Design review of the part built by this model. Coordinates are the model's own, in mm. Face numbers are marked on the shaded views. A direction names the side the tool comes from. Coordinates: 2 decimals unless noted, no trailing zeros. Write each loop counter-clockwise with the first axis right and the second up, starting at its lowest first coordinate (ties: lowest second). Pieces come first, ordered by that corner, then holes. Notation, with made-up numbers: (-20.5, 42.5) - (3.5, 42.5) arc R31 ccw to (3.5, 80.5) - close; hole circle Ø9 at (25.25, -25.75). An arc over 180 degrees is marked (long way). Answer as a JSON object with one key per item and string values.
```python
from build123d import *

# Parameters (mm, degrees)
F1_DEPTH      = 10
F1_DEPTH_BACK = 10
F2_R          = 4.5
F3_DEPTH      = 4
F4_R          = 3.5
F5_DEPTH      = 25.2476


with BuildPart() as f1:
    # F0 (on Front) → F1 (new body, two sides)
    with BuildSketch(Plane.XZ) as f1_sk:
        with BuildLine():
            ThreePointArc((4.518019, -1.1), (4.616887, -0.553945), (4.65, 0))
            ThreePointArc((4.65, 0), (4.616887, 0.553945), (4.518019, 1.1))
            ThreePointArc((4.518019, 1.1), (4.422413, 1.436929), (4.301718, 1.765707))
            ThreePointArc((4.301718, 1.765707), (3.761929, 2.733201), (3.008591, 3.545544))
            ThreePointArc((3.008591, 3.545544), (2.733201, 3.761929), (2.442307, 3.956973))
            ThreePointArc((2.442307, 3.956973), (1.436929, 4.422413), (0.349983, 4.636811))
            ThreePointArc((0.349983, 4.636811), (0, 4.65), (-0.349983, 4.636811))
            ThreePointArc((-0.349983, 4.636811), (-1.436929, 4.422413), (-2.442307, 3.956973))
            ThreePointArc((-2.442307, 3.956973), (-2.733201, 3.761929), (-3.008591, 3.545544))
            ThreePointArc((-3.008591, 3.545544), (-3.761929, 2.733201), (-4.301718, 1.765707))
            ThreePointArc((-4.301718, 1.765707), (-4.422413, 1.436929), (-4.518019, 1.1))
            ThreePointArc((-4.518019, 1.1), (-4.65, 0), (-4.518019, -1.1))
            ThreePointArc((-4.518019, -1.1), (-4.422413, -1.436929), (-4.301718, -1.765707))
            ThreePointArc((-4.301718, -1.765707), (-3.761929, -2.733201), (-3.008591, -3.545544))
            ThreePointArc((-3.008591, -3.545544), (-2.733201, -3.761929), (-2.442307, -3.956973))
            ThreePointArc((-2.442307, -3.956973), (-1.436929, -4.422413), (-0.349983, -4.636811))
            ThreePointArc((-0.349983, -4.636811), (0, -4.65), (0.349983, -4.636811))
            ThreePointArc((0.349983, -4.636811), (1.436929, -4.422413), (2.442307, -3.956973))
            ThreePointArc((2.442307, -3.956973), (2.733201, -3.761929), (3.008591, -3.545544))
            ThreePointArc((3.008591, -3.545544), (3.761929, -2.733201), (4.301718, -1.765707))
            ThreePointArc((4.301718, -1.765707), (4.422413, -1.436929), (4.518019, -1.1))
        make_face()
        with BuildLine():
            ThreePointArc((4.518019, 1.1), (4.616887, 0.553945), (4.65, 0))
            ThreePointArc((4.65, 0), (4.616887, -0.553945), (4.518019, -1.1))
            Line((4.518019, -1.1), (4.618019, -1.1))
            Line((4.618019, -1.1), (6.25, -0.329923))
            Line((6.25, -0.329923), (6.25, 0))
            Line((6.25, 0), (6.25, 0.329923))
            Line((6.25, 0.329923), (4.618019, 1.1))
            Line((4.618019, 1.1), (4.518019, 1.1))
        make_face()
        with BuildLine():
            ThreePointArc((3.008591, 3.545544), (3.761929, 2.733201), (4.301718, 1.765707))
            Line((4.301718, 1.765707), (4.38262, 1.824485))
            Line((4.38262, 1.824485), (5.25028, 3.406744))
            Line((5.25028, 3.406744), (5.056356, 3.673658))
            Line((5.056356, 3.673658), (4.862432, 3.940572))
            Line((4.862432, 3.940572), (3.089492, 3.604322))
            Line((3.089492, 3.604322), (3.008591, 3.545544))
        make_face()
        with BuildLine():
            Line((4.38262, -1.824485), (4.301718, -1.765707))
            ThreePointArc((4.301718, -1.765707), (3.761929, -2.733201), (3.008591, -3.545544))
            Line((3.008591, -3.545544), (3.089492, -3.604322))
            Line((3.089492, -3.604322), (4.862432, -3.940572))
            Line((4.862432, -3.940572), (5.056356, -3.673658))
            Line((5.056356, -3.673658), (5.25028, -3.406744))
            Line((5.25028, -3.406744), (4.38262, -1.824485))
        make_face()
        with BuildLine():
            ThreePointArc((0.349983, 4.636811), (1.436929, 4.422413), (2.442307, 3.956973))
            Line((2.442307, 3.956973), (2.473209, 4.052079))
            Line((2.473209, 4.052079), (2.245132, 5.842151))
            Line((2.245132, 5.842151), (1.931356, 5.944103))
            Line((1.931356, 5.944103), (1.61758, 6.046055))
            Line((1.61758, 6.046055), (0.380884, 4.731916))
            Line((0.380884, 4.731916), (0.349983, 4.636811))
        make_face()
        with BuildLine():
            Line((2.473209, -4.052079), (2.442307, -3.956973))
            ThreePointArc((2.442307, -3.956973), (1.436929, -4.422413), (0.349983, -4.636811))
            Line((0.349983, -4.636811), (0.380884, -4.731916))
            Line((0.380884, -4.731916), (1.61758, -6.046055))
            Line((1.61758, -6.046055), (1.931356, -5.944103))
            Line((1.931356, -5.944103), (2.245132, -5.842151))
            Line((2.245132, -5.842151), (2.473209, -4.052079))
        make_face()
        with BuildLine():
            ThreePointArc((-2.442307, 3.956973), (-1.436929, 4.422413), (-0.349983, 4.636811))
            Line((-0.349983, 4.636811), (-0.380884, 4.731916))
            Line((-0.380884, 4.731916), (-1.61758, 6.046055))
            Line((-1.61758, 6.046055), (-1.931356, 5.944103))
            Line((-1.931356, 5.944103), (-2.245132, 5.842151))
            Line((-2.245132, 5.842151), (-2.473209, 4.052079))
            Line((-2.473209, 4.052079), (-2.442307, 3.956973))
        make_face()
        with BuildLine():
            Line((-0.380884, -4.731916), (-0.349983, -4.636811))
            ThreePointArc((-0.349983, -4.636811), (-1.436929, -4.422413), (-2.442307, -3.956973))
            Line((-2.442307, -3.956973), (-2.473209, -4.052079))
            Line((-2.473209, -4.052079), (-2.245132, -5.842151))
            Line((-2.245132, -5.842151), (-1.931356, -5.944103))
            Line((-1.931356, -5.944103), (-1.61758, -6.046055))
            Line((-1.61758, -6.046055), (-0.380884, -4.731916))
        make_face()
        with BuildLine():
            ThreePointArc((-4.301718, 1.765707), (-3.761929, 2.733201), (-3.008591, 3.545544))
            Line((-3.008591, 3.545544), (-3.089492, 3.604322))
            Line((-3.089492, 3.604322), (-4.862432, 3.940572))
            Line((-4.862432, 3.940572), (-5.056356, 3.673658))
            Line((-5.056356, 3.673658), (-5.25028, 3.406744))
            Line((-5.25028, 3.406744), (-4.38262, 1.824485))
            Line((-4.38262, 1.824485), (-4.301718, 1.765707))
        make_face()
        with BuildLine():
            Line((-3.089492, -3.604322), (-3.008591, -3.545544))
            ThreePointArc((-3.008591, -3.545544), (-3.761929, -2.733201), (-4.301718, -1.765707))
            Line((-4.301718, -1.765707), (-4.38262, -1.824485))
            Line((-4.38262, -1.824485), (-5.25028, -3.406744))
            Line((-5.25028, -3.406744), (-5.056356, -3.673658))
            Line((-5.056356, -3.673658), (-4.862432, -3.940572))
            Line((-4.862432, -3.940572), (-3.089492, -3.604322))
        make_face()
        with BuildLine():
            ThreePointArc((-4.518019, -1.1), (-4.65, 0), (-4.518019, 1.1))
            Line((-4.518019, 1.1), (-4.618019, 1.1))
            Line((-4.618019, 1.1), (-6.25, 0.329923))
            Line((-6.25, 0.329923), (-6.25, 0))
            Line((-6.25, 0), (-6.25, -0.329923))
            Line((-6.25, -0.329923), (-4.618019, -1.1))
            Line((-4.618019, -1.1), (-4.518019, -1.1))
        make_face()
    extrude(amount=F1_DEPTH)
    extrude(f1_sk.sketch, amount=-F1_DEPTH_BACK)

    # F2 (on face) → F3 (join)
    with BuildSketch(Plane.XZ.offset(10)):
        Circle(F2_R)
    extrude(amount=F3_DEPTH)

    # F4 (on face) → F5 (cut)
    with BuildSketch(Plane.XZ.offset(14)):
        Circle(F4_R)
    extrude(amount=-F5_DEPTH, mode=Mode.SUBTRACT)


solid = f1.part
```
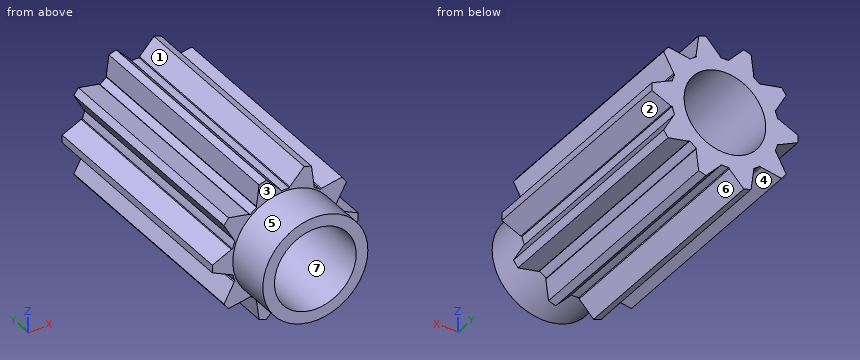
(1) The part is to be moulded in two halves that separate along Z. For the marked faces 5, 6 and 7, say which applies: pulls with the +Z half, pulls with the -Z half, needs draft (parallel to the pull), parting line crosses it, or undercut.
Solved:
{"face 5": "parting line crosses it", "face 6": "pulls with the -Z half", "face 7": "undercut"}
(2) Take a section at C-C, the plane y = -10.5. Write out the cut boundary in (x, z), and give its area (3 significant figures).
Solved:
{"outline": "circle Ø9 at (0, 0); hole circle Ø7 at (0, 0)", "area": "25.1 mm^2"}
(3) Take a section at B-B, the plane x = 0. Write out the cut boundary in (y, z).
Solved:
{"outline": "(-14, -4.5) - (-10, -4.5) - (-10, -4.65) - (10, -4.65) - (10, -3.5) - (-14, -3.5) - close; (-14, 3.5) - (10, 3.5) - (10, 4.65) - (-10, 4.65) - (-10, 4.5) - (-14, 4.5) - close"}
(4) Tool access review of the marked faces 1, 2, 3 and 4: name each direction out of +Z, -Z, +X, -X, +Y, -Y from which nothing blocks a thin tool from reaching the whole face with its end or side.
Solved:
{"face 1": "+Z, +Y, -Y", "face 2": "+X, +Y, -Y", "face 3": "-Y", "face 4": "-Z, +Y, -Y"}
(5) To check wall thickness, follow line 1 (X direction, y = -7.75, z = 0.25); line 2 (Z direction, x = -1.25, y = -12); line 3 (Z direction, x = 2.75, y = 3.5). State the ranges of each line that lie inside material, in increasing order. Write a range as from..to.
Solved:
{"line 1": "x = -6.25..-3.49, 3.49..6.25", "line 2": "z = -4.32..-3.27, 3.27..4.32", "line 3": "z = -3.75..-2.17, 2.17..3.75"}
(6) Take a section at A-A, the plane z = 0. Write out the cut boundary in (x, y), and give its area (3 significant figures).
Solved:
{"outline": "(-6.25, -10) - (-4.5, -10) - (-4.5, -14) - (-3.5, -14) - (-3.5, 10) - (-6.25, 10) - close; (3.5, -14) - (4.5, -14) - (4.5, -10) - (6.25, -10) - (6.25, 10) - (3.5, 10) - close", "area": "118 mm^2"}
